Input: part model. Units: mm. Frame: model coordinates. A direction names the side the tool comes from. Round coordinates to 2 decimals unless told otherwise and drop trailing zeros. Loops run counter-clockwise (first coordinate to the right, second up) from the corner with the lowest first, then second, coordinate; pieces in that order, holes last. Notation, with made-up numbers: M 84,11 L 91,11 A33 ccw 91,48 Z; hole C 73,-28.5 d7. An arc over 180 degrees is marked long. Use one line per item in the form item = value. Start each with the question number.
Q1. Mould query, pull axis X, two halves, no side actions, for faces 4 (the flat face through (10, -9, 0)), 5 (the flat face through (-10, 0, 0)), 6 (the flat face through (0, -10, 0)), 7 (the cylindrical face through (-0.57, -8.52, -12.59)). Classes: pulls with the +X half, pulls with the -X half, needs draft (parallel to the pull), parting line crosses it, or undercut.
Q2. First-contact query: P1, Ø9.5, axis at y = 0, z = 10, coming from the +X side; P2, Ø2, axis at x = -1.5, z = -2, coming from the +Y side; P3, Ø10.5, axis at y = 2, z = -4, coming from the +X side. Flat tips, straight axial feed; report the tip coordinate or a pass-through.
Q3. Section query D-D, the plane x = -4. Output: boundary loops of the cut face in (y, z).
Q4. Section query A-A, the plane z = 10. Output: boundary loops of the cut face in (x, y).
Q5. Access query for faces 1 (the flat face through (-8, 10, 0)), 2 (the cylindrical face through (6.32, -5.95, -10.76)), 3 (the cylindrical face through (-5.95, 6.32, 10.76)). Directions: +Z, -Z, +X, -X, +Y, -Y. A direction counts if a zero-diameter tool reaches every point of the face in a straight line with its end or side. Return the directions, or none.
Q6. Section query B-B, the plane x = -1.5. Output: boundary loops of the cut face in (y, z), and give its area (3 significant figures).
Q7. Section query C-C, the plane z = -2.5. Output: boundary loops of the cut face in (x, y), and give its area (3 significant figures).
Q8. Ray query, line 1 along Z through (x, y) = (0, 2.5); line 2 along Z through (x, y) = (-9.1, 0); line 3 along X through (y, z) = (-6.5, 0). Return the intervals inside material, ascending.
```python
from build123d import *

# Parameters (mm, degrees)
BOSS_EXTRUDE1_DEPTH     = 18.5
SKETCH4_R               = 2.65
CUT_EXTRUDE1_DEPTH      = 3
SKETCH6_R               = 6
CUT_EXTRUDE2_DEPTH      = 18
MIRROR2_COPY_1_SKETCH_R = 2.65
MIRROR2_COPY_1_DEPTH    = 3
MIRROR2_COPY_2_SKETCH_R = 6
MIRROR2_COPY_2_DEPTH    = 18
MIRROR2_COPY_3_SKETCH_R = 2.65
MIRROR2_COPY_3_DEPTH    = 3


with BuildPart() as part:
    # Sketch2 → Boss-Extrude1 (new body, symmetric)
    with BuildSketch(Plane.XY):
        Polygon((-10, 10), (-10, -10), (10, -10), (10, -7), (-7, 10), align=None)
        Polygon((-7, 5.757359313), (-7, -7), (5.757359313, -7), align=None, mode=Mode.SUBTRACT)
    extrude(amount=BOSS_EXTRUDE1_DEPTH, both=True)

    # Sketch4 → Cut-Extrude1 (cut)
    with BuildSketch(Plane.XZ.offset(10)):
        with Locations((0, -10)):
            Circle(SKETCH4_R)
        with Locations((0, 10)):
            Circle(SKETCH4_R)
    cut_extrude1 = extrude(amount=-CUT_EXTRUDE1_DEPTH, mode=Mode.SUBTRACT)

    # Sketch6 → Cut-Extrude2 (cut, through all)
    with BuildSketch(Plane(origin=(0, -7, 0), x_dir=(1, 0, 0), z_dir=(0, 1, 0))):
        with Locations((0, -10)):
            Circle(SKETCH6_R)
    cut_extrude2 = extrude(amount=CUT_EXTRUDE2_DEPTH, mode=Mode.SUBTRACT)

    # Mirror1: Cut-Extrude1, Cut-Extrude2 across plane
    add(cut_extrude1.mirror(Plane(origin=(0, 0, 0), x_dir=(0, 0, 1), z_dir=(0.707106781, -0.707106781, 0))), mode=Mode.SUBTRACT)
    add(cut_extrude2.mirror(Plane(origin=(0, 0, 0), x_dir=(0, 0, 1), z_dir=(0.707106781, -0.707106781, 0))), mode=Mode.SUBTRACT)

    # Mirror2: Cut-Extrude2 across plane
    add(cut_extrude2.mirror(Plane.XY), mode=Mode.SUBTRACT)

    # Mirror2 copy 1 sketch → Mirror2 copy 1 (cut)
    with BuildSketch(Plane(origin=(-10, 0, 0), x_dir=(0, 1, 0), z_dir=(-1, 0, 0))):
        with Locations((0, -10)):
            Circle(MIRROR2_COPY_1_SKETCH_R)
        with Locations((0, 10)):
            Circle(MIRROR2_COPY_1_SKETCH_R)
    extrude(amount=-MIRROR2_COPY_1_DEPTH, mode=Mode.SUBTRACT)

    # Mirror2 copy 2 sketch → Mirror2 copy 2 (cut, through all)
    with BuildSketch(Plane.YZ.offset(-7)):
        with Locations((0, -10)):
            Circle(MIRROR2_COPY_2_SKETCH_R)
    extrude(amount=MIRROR2_COPY_2_DEPTH, mode=Mode.SUBTRACT)

    # Mirror2 copy 3 sketch → Mirror2 copy 3 (cut)
    with BuildSketch(Plane.XZ.offset(10)):
        with Locations((0, 10)):
            Circle(MIRROR2_COPY_3_SKETCH_R)
        with Locations((0, -10)):
            Circle(MIRROR2_COPY_3_SKETCH_R)
    extrude(amount=-MIRROR2_COPY_3_DEPTH, mode=Mode.SUBTRACT)


solid = part.part
```
Results found:
q1.face_4 = pulls with the +X half
q1.face_5 = pulls with the -X half
q1.face_6 = needs draft
q1.face_7 = undercut
q2.P1 = -7
q2.P2 = 5.5
q2.P3 = 6.25
q3.outline = M -10,-18.5 L -7,-18.5 L -7,18.5 L -10,18.5 Z; M 2.76,-18.5 L 7,-18.5 L 7,-14.47 L 4,-14.47 A6 cw 2.76,-15.33 Z; M 2.76,-4.67 A6 cw 4,-5.53 L 7,-5.53 L 7,5.53 L 4,5.53 A6 cw 2.76,4.67 Z; M 2.76,15.33 A6 cw 4,14.47 L 7,14.47 L 7,18.5 L 2.76,18.5 Z
q4.outline = M -10,-10 L -2.65,-10 L -2.65,-7 L -7,-7 L -7,-2.65 L -10,-2.65 Z; M -10,2.65 L -7,2.65 L -7,6 L -6,6 L -6,9 L -7,10 L -10,10 Z; M 2.65,-10 L 10,-10 L 10,-7 L 9,-6 L 6,-6 L 6,-7 L 2.65,-7 Z
q5.face_1 = +Z, -Z, +X, -X, +Y
q5.face_2 = +X
q5.face_3 = +Y
q6.outline = M -10,-18.5 L -7,-18.5 L -7,-12.18 L -10,-12.18 Z; M -10,-7.82 L -7,-7.82 L -7,7.82 L -10,7.82 Z; M -10,12.18 L -7,12.18 L -7,18.5 L -10,18.5 Z; M 0.26,-18.5 L 4.5,-18.5 L 4.5,-15.81 L 1.5,-15.81 A6 cw 0.26,-15.99 Z; M 0.26,-4.01 A6 cw 1.5,-4.19 L 4.5,-4.19 L 4.5,4.19 L 1.5,4.19 A6 cw 0.26,4.01 Z; M 0.26,15.99 A6 cw 1.5,15.81 L 4.5,15.81 L 4.5,18.5 L 0.26,18.5 Z
q6.area = 143 mm²
q7.outline = M -10,-10 L 10,-10 L 10,-7 L -7,10 L -10,10 Z; hole M -7,-7 L 5.76,-7 L -7,5.76 Z
q7.area = 174 mm²
q8.line_1 = -18.5 to -16, -4 to 4, 16 to 18.5
q8.line_2 = -18.5 to -12.65, -7.35 to 7.35, 12.65 to 18.5
q8.line_3 = -10 to -7, 5.26 to 9.5
